```python
from build123d import *

# Parameters (mm, degrees)
F1_DEPTH = 70
F2_W     = 53
F2_H     = 53
F3_DEPTH = 50
F4_R     = 5
F5_R     = 12.5
F6_DEPTH = 90
F7_SIZE  = 1


with BuildPart() as f1:
    # F0 (on Top) → F1 (new body)
    with BuildSketch(Plane.XY):
        with BuildLine():
            ThreePointArc((-60, 3.2), (-59.062742, 0.937258), (-56.8, 0))
            Line((-56.8, 0), (-3.2, 0))
            ThreePointArc((-3.2, 0), (-0.937258, 0.937258), (0, 3.2))
            Line((0, 3.2), (0, 56.8))
            ThreePointArc((0, 56.8), (-0.937258, 59.062742), (-3.2, 60))
            Line((-3.2, 60), (-56.8, 60))
            ThreePointArc((-56.8, 60), (-59.062742, 59.062742), (-60, 56.8))
            Line((-60, 56.8), (-60, 3.2))
        make_face()
    extrude(amount=F1_DEPTH)

    # F2 (on face) → F3 (cut)
    with BuildSketch(Plane(origin=(0, 0, 0), x_dir=(1, 0, 0), z_dir=(0, 0, -1))):
        with BuildLine():
            Line((-3.2, 0), (-56.8, 0))
            ThreePointArc((-56.8, 0), (-59.062742, -0.937258), (-60, -3.2))
            Line((-60, -3.2), (-60, -56.8))
            ThreePointArc((-60, -56.8), (-59.062742, -59.062742), (-56.8, -60))
            Line((-56.8, -60), (-3.2, -60))
            ThreePointArc((-3.2, -60), (-0.937258, -59.062742), (0, -56.8))
            Line((0, -56.8), (0, -3.2))
            ThreePointArc((0, -3.2), (-0.937258, -0.937258), (-3.2, 0))
        make_face()
        with Locations((-30, -30)):
            Rectangle(F2_W, F2_H, mode=Mode.SUBTRACT)
    extrude(amount=-F3_DEPTH, mode=Mode.SUBTRACT)

    # F4
    f4_edges = [f1.edges().sort_by_distance(p)[0] for p in [
        (-56.5, 3.5, 25),
        (-3.5, 3.5, 25),
        (-3.5, 56.5, 25),
        (-56.5, 56.5, 25),
    ]]
    fillet(f4_edges, radius=F4_R)

    # F5 (on face) → F6 (join)
    with BuildSketch(Plane.XY.offset(70)):
        with Locations((-30, 30)):
            Circle(F5_R)
    extrude(amount=F6_DEPTH)

    # F7
    f7_edges = [f1.edges().sort_by_distance(p)[0] for p in [
        (-42.5, 30, 160),
    ]]
    chamfer(f7_edges, length=F7_SIZE)


solid = f1.part
```
Geometry check sheet. Reference: the model listing, model coordinates, mm. A direction names the side the tool comes from. Give positions to 0.01 mm unless a question says otherwise; leave off trailing zeros. Write each loop counter-clockwise with the first axis right and the second up, starting at its lowest first coordinate (ties: lowest second). Pieces come first, ordered by that corner, then holes. Notation, with made-up numbers: (30.25, 77) - (38.25, 77) arc R25 ccw to (38.25, 89) - close; hole circle Ø8 at (-30, 63). An arc over 180 degrees is marked (long way). Use a Markdown table: item, result.
Q1. Set-up check for faces 1 (the face through (-3.5, 30, 25)), 2 (the face through (-55, 4.93, 25.35)), 3 (the face through (-39.21, 38.45, 113.88)): record each of +Z, -Z, +X, -X, +Y, -Y from which the full face is reachable in a straight line by a thin tool's end or side.
Computed:
| item | result |
|---|---|
| face 1 | -Z, +X, +Y, -Y |
| face 2 | -Z, -X, -Y |
| face 3 | +Z |
Q2. Section check C-C, the plane z = 143. Enter the section's corners in (x, y).
Computed:
| item | result |
|---|---|
| outline | circle Ø25 at (-30, 30) |
Q3. Thickness scan on L1, parallel to Y at x = -30, z = 109.5; L2, parallel to Z at x = -10.5, y = 41.5; L3, parallel to X at y = 36, z = 34.5. Record the ranges inside material, lowest first. Write a range as [from, to].
Computed:
| item | result |
|---|---|
| L1 | y = [17.5, 42.5] |
| L2 | z = [0, 70] |
| L3 | x = [-56.5, -3.5] |
Q4. Go/stop test with flat-tipped pins: P1, Ø1.5, axis at x = -27.5, y = 6.5, coming from the +Z side; P2, Ø5, axis at y = 28.5, z = 76, coming from the -X side; P3, Ø13, axis at x = -25.5, z = 34, coming from the +Y side. Record where each tip stops, or that it passes through.
Computed:
| item | result |
|---|---|
| P1 | stops at z = 70 |
| P2 | stops at x = -42.5 |
| P3 | stops at y = 56.5 |
Q5. Section check B-B, the plane y = 12. Enter the section's corners in (x, z), then the cut area to 3 significant figures.
Computed:
| item | result |
|---|---|
| outline | (-60, 50) - (-56.5, 50) - (-56.5, 0) - (-3.5, 0) - (-3.5, 50) - (0, 50) - (0, 70) - (-60, 70) - close |
| area | 3,850 mm² |
Q6. Section check D-D, the plane x = -12.5. Enter the section's corners in (y, z), then the cut area to 3 significant figures.
Computed:
| item | result |
|---|---|
| outline | (0, 50) - (3.5, 50) - (3.5, 0) - (56.5, 0) - (56.5, 50) - (60, 50) - (60, 70) - (0, 70) - close |
| area | 3,850 mm² |
Q7. Section check A-A, the plane x = -30. Enter the section's corners in (y, z), then the cut area to 3 significant figures.
Computed:
| item | result |
|---|---|
| outline | (0, 50) - (3.5, 50) - (3.5, 0) - (56.5, 0) - (56.5, 50) - (60, 50) - (60, 70) - (42.5, 70) - (42.5, 159) - (41.5, 160) - (18.5, 160) - (17.5, 159) - (17.5, 70) - (0, 70) - close |
| area | 6,100 mm² |
